from build123d import *

# Parameters (mm, degrees)
SKETCH1_W               = 28.5
SKETCH1_H               = 23
CENTRE_BLOCK_DEPTH      = 128
TOP_CYLINDER_DEPTH      = 7
TOP_CYLINDER_DEPTH_BACK = 90
CUT_REVOLVE2_ANGLE      = 180
NOSE_DEPTH              = 131.828370394
T_CROSS_REACH           = 134.885
SKETCH6_R               = 12
BARREL_DEPTH            = 7
SIDE_CYLINDER_DEPTH     = 128
CUT_REVOLVE1_ANGLE      = 180
SKETCH8_R               = 2.75
BACK_HOLE_DEPTH         = 5
SKETCH12_W              = 5
SKETCH12_H              = 80
CUT_EXTRUDE4_DEPTH      = 5
SKETCH15_R              = 2.75
CUT_EXTRUDE6_DEPTH      = 10
FILLET2_R               = 1
SKETCH16_R              = 6.5
CUT_EXTRUDE7_DEPTH      = 20
SKETCH21_W              = 152.585030794
SKETCH21_H              = 42.838852891
CUT_EXTRUDE12_DEPTH     = 133.885289011
SKETCH24_R              = 2.75
CUT_EXTRUDE13_DEPTH     = 5


with BuildPart() as part:
    # Sketch1 → Centre block (new body)
    with BuildSketch(Plane.XY):
        Rectangle(SKETCH1_W, SKETCH1_H)
    extrude(amount=CENTRE_BLOCK_DEPTH)

    # Sketch3 → top cylinder (add, two sides: drawn at the far end of the back side and taken through both)
    with BuildSketch(Plane(origin=(0, 0, 0), x_dir=(-1, 0, 0), z_dir=(0, 0, -1)).offset(-TOP_CYLINDER_DEPTH_BACK)):
        with BuildLine():
            Line((-10, 11.5), (10, 11.5))
            ThreePointArc((10, 11.5), (0, 21.5), (-10, 11.5))
        make_face()
    extrude(amount=TOP_CYLINDER_DEPTH + TOP_CYLINDER_DEPTH_BACK)

    # Sketch9 → Cut-Revolve2 (revolve, cut)
    with BuildSketch(Plane(origin=(0, 11.5, 0), x_dir=(1, 0, 0), z_dir=(0, 1, 0))):
        Polygon((10, -78), (10, -81.888582416), (23.187071127, -81.888582416), (23.187071127, -74.052631606), (23.187071127, 0), (10, 0), (10, -8), (9.5, -8), (9.5, -8.5), (10, -8.5), (10, -11.5), (8, -13.5), (8, -16.5), (10, -18.5), (10, -21.5), (9.5, -21.5), (9.5, -22), (10, -22), (10, -25), (9.5, -25), (9.5, -25.5), (10, -25.5), (10, -28.5), (8, -30.5), (8, -33.5), (10, -35.5), (10, -38.5), (8, -38.5), (8, -41.5), (10, -43.5), (10, -48.5), (8, -48.5), (8, -51.5), (10, -53.5), (10, -58.5), (8, -58.5), (8, -60.3), (8, -61.5), (10, -63.5), (10, -68.5), (8, -68.5), (8, -70.3), (8, -71.5), (10, -73.5), (10, -74.052631606), (10, -77.5), (9.5, -77.5), (9.5, -78), align=None)
    revolve(axis=Axis((0, 11.5, -7), (0, 0, 1)), revolution_arc=CUT_REVOLVE2_ANGLE, mode=Mode.SUBTRACT)

    # Sketch4 → nose (cut, through all)
    with BuildSketch(Plane.XZ.offset(-11.5)):
        with BuildLine():
            Line((-3.25, -7), (-3.25, -2))
            ThreePointArc((-3.25, -2), (-3.835786438, -0.585786438), (-5.25, 0))
            Line((-5.25, 0), (-10, 0))
            Line((-10, 0), (-10, -7))
            Line((-10, -7), (-3.25, -7))
        make_face()
        with BuildLine():
            Line((3.75, -7), (3.75, -2))
            ThreePointArc((3.75, -2), (4.335786438, -0.585786438), (5.75, 0))
            Line((5.75, 0), (10, 0))
            Line((10, 0), (10, -7))
            Line((10, -7), (3.75, -7))
        make_face()
    extrude(amount=-NOSE_DEPTH, mode=Mode.SUBTRACT)

    # t cross: up to this face of the body (flat: up to its plane)
    t_cross_end = Plane(part.part.faces().sort_by_distance((-14.25, 0, 64))[0])
    # Sketch5 → t cross (add, up to the picked face)
    with BuildSketch(Plane(origin=(14.25, 0, 0), x_dir=(0, 0, -1), z_dir=(1, 0, 0)), mode=Mode.PRIVATE) as t_cross_sk1:
        with BuildLine():
            Line((-101, 11.5), (-81, 11.5))
            ThreePointArc((-81, 11.5), (-91, 21.5), (-101, 11.5))
        make_face()
    t_cross_tool1 = split(extrude(t_cross_sk1.sketch, amount=-T_CROSS_REACH, mode=Mode.PRIVATE), bisect_by=t_cross_end, keep=Keep.BOTH, mode=Mode.PRIVATE)
    add(t_cross_tool1.solids().sort_by(Axis((14.25, 15.744132, 91), (-1, 0, 0)))[0])

    # Sketch6 → Barrel (add)
    with BuildSketch(Plane(origin=(0, 0, 0), x_dir=(-1, 0, 0), z_dir=(0, 0, -1))):
        with Locations((0, 0.5)):
            Circle(SKETCH6_R)
    extrude(amount=BARREL_DEPTH)

    # Sketch2 → side cylinder (add)
    with BuildSketch(Plane(origin=(0, 0, 0), x_dir=(-1, 0, 0), z_dir=(0, 0, -1))):
        with BuildLine():
            Line((14.25, 10), (14.25, -10))
            ThreePointArc((14.25, -10), (24.25, 0), (14.25, 10))
        make_face()
    extrude(amount=-SIDE_CYLINDER_DEPTH)

    # Sketch7 → Cut-Revolve1 (revolve, cut)
    with BuildSketch(Plane(origin=(-14.25, 0, 0), x_dir=(0, 0, -1), z_dir=(1, 0, 0))):
        Polygon((-51, -10), (-51, -9), (-51.5, -9), (-51.5, -10), (-55.5, -10), (-57.5, -8), (-58.77482941, -8), (-60.5, -8), (-60.5, -10), (-64.5, -10), (-66.5, -8), (-67.77482941, -8), (-69.5, -8), (-69.5, -10), (-73.5, -10), (-75.5, -8), (-76.77482941, -8), (-78.5, -8), (-78.5, -10), (-82.5, -10), (-84.5, -8), (-85.77482941, -8), (-87.5, -8), (-87.5, -10), (-91.5, -10), (-93.5, -8), (-94.77482941, -8), (-96.5, -8), (-96.5, -10), (-100.5, -10), (-102.5, -8), (-105.5, -8), (-107.5, -10), (-110.5, -10), (-110.5, -9), (-111, -9), (-111, -10), (-114, -10), (-114, -9), (-114.5, -9), (-114.5, -10), (-117.5, -10), (-119.5, -8), (-122.65, -8), (-124.65, -10), (-124.65, -14.812383498), (-117.5, -14.812383498), (0, -14.812383498), (0, -10), align=None)
    revolve(axis=Axis((-14.25, 0, 135.382259058), (0, 0, -1)), revolution_arc=CUT_REVOLVE1_ANGLE, mode=Mode.SUBTRACT)

    # Sketch8 → Back hole (cut)
    with BuildSketch(Plane.XY.offset(128)):
        Circle(SKETCH8_R)
    extrude(amount=-BACK_HOLE_DEPTH, mode=Mode.SUBTRACT)

    # Sketch12 → Cut-Extrude4 (cut)
    with BuildSketch(Plane.XZ.offset(11.5)):
        with Locations((0, 78)):
            Rectangle(SKETCH12_W, SKETCH12_H)
    extrude(amount=-CUT_EXTRUDE4_DEPTH, mode=Mode.SUBTRACT)

    # Sketch15 → Cut-Extrude6 (cut)
    with BuildSketch(Plane(origin=(14.25, 0, 0), x_dir=(0, 0, -1), z_dir=(1, 0, 0))):
        with Locations((-91, 11.5)):
            Circle(SKETCH15_R)
        with Locations((-91, -5.5)):
            Circle(SKETCH15_R)
    extrude(amount=-CUT_EXTRUDE6_DEPTH, mode=Mode.SUBTRACT)

    # Fillet2
    fillet2_edges = [part.edges().sort_by_distance(p)[0] for p in [
        (-14.25, 11.5, 40.5),
        (14.25, 11.5, 40.5),
        (14.25, -11.5, 64),
        (-14.25, -11.5, 64),
        (-14.25, 11.5, 114.5),
        (14.25, 11.5, 114.5),
    ]]
    fillet(fillet2_edges, radius=FILLET2_R)

    # Sketch16 → Cut-Extrude7 (cut)
    with BuildSketch(Plane(origin=(0, 0, -7), x_dir=(-1, 0, 0), z_dir=(0, 0, -1))):
        Circle(SKETCH16_R)
    extrude(amount=-CUT_EXTRUDE7_DEPTH, mode=Mode.SUBTRACT)

    # Sketch21 → Cut-Extrude12 (cut, through all)
    with BuildSketch(Plane.ZY.offset(14.25)):
        with Locations((64.09795532, 3.365381731)):
            Rectangle(SKETCH21_W, SKETCH21_H)
    extrude(amount=-CUT_EXTRUDE12_DEPTH, mode=Mode.SUBTRACT)

    # Sketch24 → Cut-Extrude13 (cut)
    with BuildSketch(Plane(origin=(-14.25, 0, 0), x_dir=(0, 0, -1), z_dir=(1, 0, 0))):
        with Locations((-118, 0)):
            Circle(SKETCH24_R)
        with Locations((-64, 0)):
            Circle(SKETCH24_R)
        with Locations((-10, 0)):
            Circle(SKETCH24_R)
    extrude(amount=-CUT_EXTRUDE13_DEPTH, mode=Mode.SUBTRACT)


solid = part.part
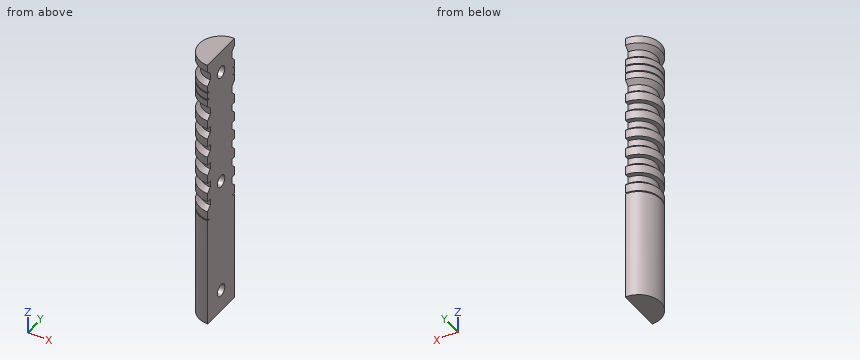
Source: CAD feature listing. Evaluate the final solid. Frame: model axes, mm. Round coordinates to 2 decimals unless told otherwise and drop trailing zeros. Loops run counter-clockwise (first coordinate to the right, second up) from the corner with the lowest first, then second, coordinate; pieces in that order, holes last. Notation, with made-up numbers: M 41.25,-34.5 L 66.25,-34.5 A16 cw 66.25,-19.5 Z; hole C 89.5,65.5 d10. An arc over 180 degrees is marked long. Return JSON: item names as keys, results as strings. Group by question number.
1. Section query B-B on x = -16.5. State how many separate pieces and enclosed holes the cut face has, and give its area (3 significant figures).
2. Pin query (flat end, axial travel): pin 1 (1.6 mm diameter, centred on y = 1, z = 65, fed in from +X); pin 2 (2 mm diameter, centred on x = -16.5, z = 104, fed in from +Y); pin 3 (6 mm diameter, centred on x = -18, z = 21.5, fed in from -Y). Return the tip coordinate at first contact, or that it passes through.
3. Material intervals for line 1 along Y through (x, z) = (-16.05, 118); line 2 along Y through (x, z) = (-16.05, 10); line 3 along Y through (x, z) = (-14.75, 102.5), sorted ascending. Write a range as from..to.
4. Section query A-A on z = 11.5. Output: boundary loops of the cut face in (x, y).
Checks:
{
 "1": {"separate pieces": "1", "enclosed holes": "3", "area": "2,300 mm²"},
 "2": {"pin 1": "stops at x = -19.25", "pin 2": "stops at y = 7.9", "pin 3": "stops at y = -9.97"},
 "3": {"line 1": "y = -9.33..-2.75, 2.75..9.33", "line 2": "y = -9.84..-2.75, 2.75..9.84", "line 3": "y = -7.98..7.98"},
 "4": {"outline": "M -19.25,-2.3 L -19.25,2.3 L -14.25,2.3 L -14.25,10 A10 ccw -14.25,-10 L -14.25,-2.3 Z"}
}
